from build123d import *

# Parameters (mm, degrees)
SKETCH1_W           = 228.6
SKETCH1_H           = 49.499999806
BOSS_EXTRUDE1_DEPTH = 4.599999944
SKETCH3_W           = 25.4
SKETCH3_H           = 4.599999944
CUT_EXTRUDE1_DEPTH  = 234.943091328
SKETCH4_W           = 4.599999944
SKETCH4_H           = 40.299999918
CUT_EXTRUDE2_DEPTH  = 234.943091328


with BuildPart() as part:
    # Sketch1 → Boss-Extrude1 (new body)
    with BuildSketch(Plane(origin=(0, 0, 0), x_dir=(1, 0, 0), z_dir=(0, 1, 0))):
        with Locations((114.3, 24.749999903)):
            Rectangle(SKETCH1_W, SKETCH1_H)
    extrude(amount=BOSS_EXTRUDE1_DEPTH)

    # Sketch3 → Cut-Extrude1 (cut, through all)
    with BuildSketch(Plane(origin=(0, 4.599999944, 0), x_dir=(1, 0, 0), z_dir=(0, 1, 0))):
        with Locations((12.7, 2.299999972)):
            Rectangle(SKETCH3_W, SKETCH3_H)
        with Locations((63.5, 2.299999972)):
            Rectangle(SKETCH3_W, SKETCH3_H)
        with Locations((114.3, 2.299999972)):
            Rectangle(SKETCH3_W, SKETCH3_H)
        with Locations((165.1, 2.299999972)):
            Rectangle(SKETCH3_W, SKETCH3_H)
        with Locations((215.9, 2.299999972)):
            Rectangle(SKETCH3_W, SKETCH3_H)
    cut_extrude1 = extrude(amount=-CUT_EXTRUDE1_DEPTH, mode=Mode.SUBTRACT)

    # Mirror1: Cut-Extrude1 across plane
    add(cut_extrude1.mirror(Plane(origin=(0, 0, -24.749999903), x_dir=(1, 0, 0), z_dir=(0, 0, -1))), mode=Mode.SUBTRACT)

    # Sketch4 → Cut-Extrude2 (cut, through all)
    with BuildSketch(Plane(origin=(0, 4.599999944, 0), x_dir=(1, 0, 0), z_dir=(0, 1, 0))):
        with Locations((2.299999972, 24.749999903)):
            Rectangle(SKETCH4_W, SKETCH4_H)
    extrude(amount=-CUT_EXTRUDE2_DEPTH, mode=Mode.SUBTRACT)


solid = part.part
Work out the finished part from the listing and answer in its coordinate system (mm). A direction names the side the tool comes from. Give positions to 0.01 mm unless a question says otherwise; leave off trailing zeros. Loops run counter-clockwise (first coordinate to the right, second up) from the corner with the lowest first, then second, coordinate; pieces in that order, holes last. Notation, with made-up numbers: (10, 83.25) - (62, 83.25) arc R22 ccw to (62, 101.25) - close; hole circle Ø8 at (-14, 57). An arc over 180 degrees is marked (long way). Answer in a Markdown table with one row per item.
(1) Consider L1, parallel to X at y = 3.3, z = -3.5; L2, parallel to Z at x = 210, y = 0.55. Determine where each line is inside the solid, lowest interval first. Write a range as [from, to].
Results list:
| item | result |
|---|---|
| L1 | x = [25.4, 50.8], [76.2, 101.6], [127, 152.4], [177.8, 203.2] |
| L2 | z = [-44.9, -4.6] |
(2) A tool of negligible diameter and unlimited length cuts with its end or side. For faces 1 (the face through (15, 2, -44.9)), 2 (the face through (190, 2, -49.5)), 3 (the face through (216, 2, -44.9)), 4 (the face through (127, 2, -2)), 5 (the face through (165, 2, -44.9)), from which of +Z, -Z, +X, -X, +Y, -Y can it reach the whole face along a straight path? Write none if from no direction.
Results list:
| item | result |
|---|---|
| face 1 | -Z, -X, +Y, -Y |
| face 2 | -Z, +X, -X, +Y, -Y |
| face 3 | -Z, +X, +Y, -Y |
| face 4 | +Z, +Y, -Y |
| face 5 | -Z, +Y, -Y |
(3) Flat-ended cylindrical pins translate along their axes: pin 1 Ø2.5 at (y, z) = (1, -47.5) entering from +X; pin 2 Ø2.5 at (y, z) = (2, -2) entering from -X; pin 3 Ø2.5 at (x, y) = (160, 3.5) entering from +Z. Find the tip coordinate at first contact, or state that the pin passes through.
Results list:
| item | result |
|---|---|
| pin 1 | stops at x = 203.2 |
| pin 2 | stops at x = 25.4 |
| pin 3 | stops at z = -4.6 |
(4) Section A-A (x = 115.5) is taken. Give the vertices of the cut face in (y, z).
Results list:
| item | result |
|---|---|
| outline | (0, -44.9) - (4.6, -44.9) - (4.6, -4.6) - (0, -4.6) - close |
(5) For a pull along X with two mould halves and no side action, classify faces 6 (the face through (115, 0, -25)), 7 (the face through (203.2, 2, -47)), 8 (the face through (76.2, 2, -2)) as pulls with the +X half, pulls with the -X half, needs draft (parallel to the pull), parting line crosses it, or undercut.
Results list:
| item | result |
|---|---|
| face 6 | needs draft |
| face 7 | pulls with the +X half |
| face 8 | undercut |
